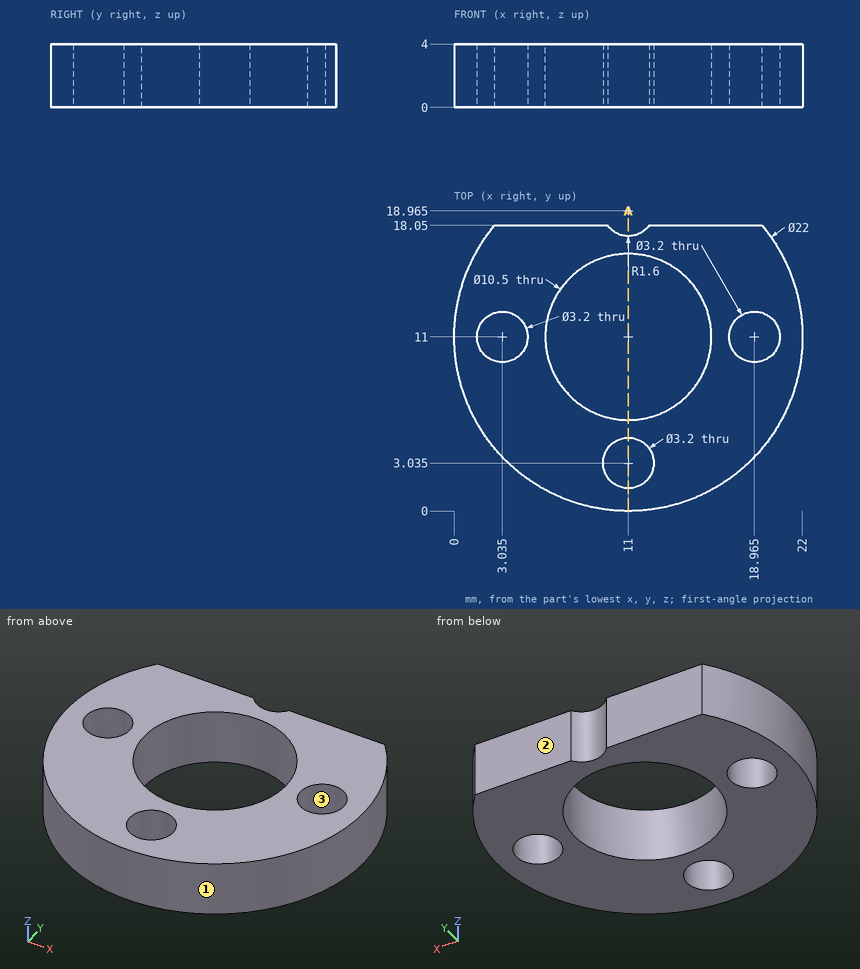
Job drawing, mm, ordinate dimensions from the low corner. One solid piece. Coordinates: 2 decimals unless noted, no trailing zeros. Return JSON: item names as keys, results as strings. Group by question number.
1) Probe line 1 (X direction, y = 10.25, z = 2.35) (1 decimal); line 2 (X direction, y = 14, z = 2.2); line 3 (Y direction, x = 12.25, z = 1.2) (1 decimal). List the from-to ranges inside material, lowest first. Write a range as from..to.
2) Mould opens along X. For the marked faces 1, 2 and 3 say: released by +X, released by -X, zero draft, split by the parting line, or undercut.
3) Flat gauge pin, fed straight in: P1, Ø1.9, axis at x = 11, y = 3.04, coming from the +Z side. Where does the tip first touch, or does it go through?
4) Saw through at A-A, the plane x = 11. Count the separate pieces of the cut face and the enclosed holes in it.
Values found:
{
 "1": {"line 1": "x = 0..1.6, 4.4..5.8, 16.2..17.6, 20.4..22", "line 2": "x = 0.42..6.69, 15.31..21.58", "line 3": "y = 0.1..2, 4..5.9, 16.1..18"},
 "2": {"face 1": "split by the parting line", "face 2": "zero draft", "face 3": "undercut"},
 "3": {"P1": "passes through"},
 "4": {"separate pieces": "3", "enclosed holes": "0"}
}
